Input: part model. Units: mm. Frame: model coordinates. A direction names the side the tool comes from. Give positions to 0.01 mm unless a question says otherwise; leave off trailing zeros. Order: outer loops, then holes, each group sorted by start corner. A loop starts at its lowest first (then second) coordinate and runs counter-clockwise, first axis right, second up. Notation, with made-up numbers: (15, 39.5) - (31, 39.5) arc R33 ccw to (31, 67.5) - close; hole circle Ø3 at (40, -6.75). An arc over 180 degrees is marked (long way). Answer in a Markdown table with one row per item. Add a question column.
1. Mould query, pull axis Y, two halves, no side actions, for faces 3 (the face through (-2, 2, 0)), 4 (the face through (69.59, 102.26, -3.04)), 5 (the face through (-2, -130, -3)). Classes: released by +Y, released by -Y, zero draft, split by the parting line, or undercut.
2. Access query for faces 1 (the face through (-132.5, -2, -3)), 2 (the face through (75, 109.05, -3)). Directions: +Z, -Z, +X, -X, +Y, -Y. A direction counts if a zero-diameter tool reaches every point of the face in a straight line with its end or side. Return the directions, or none.
3. Ray query, line 1 (X direction, y = -78, z = -3.65) (3 decimals); line 2 (Y direction, x = -99.65, z = -3.5); line 3 (Y direction, x = -49, z = -5.2). Return the intervals inside material, ascending. Write a range as [from, to].
4. Section query B-B on z = -3.25. Count the separate pieces of the cut face and the enclosed holes in it, and give its area (3 significant figures).
5. Section query A-A on x = -99.65. Return loops of the section in (y, z).
```python
from build123d import *

# Parameters (mm, degrees)
CROQUIS1_W                        = 265
CROQUIS1_H                        = 260
BRIDA_BASE1_DEPTH                 = 6
TALADRO_DE_MARGEN_PARA_M181_D     = 20
DI_METRO_DE_TALADRO_16_0_16_1_D   = 16
RANURA_START                      = -6
RANURA_DE_MARGEN_PARA_M3_54_DEPTH = 6
TALADRO_DE_MARGEN_PARA_M31_D      = 3.75
CORTAR_EXTRUIR1_DEPTH             = 186.72089274
CORTAR_EXTRUIR1_DEPTH_BACK        = 186.72089274
CROQUIS23_R                       = 1.875
CORTAR_EXTRUIR3_DEPTH             = 186.72089274
CORTAR_EXTRUIR3_DEPTH_BACK        = 186.72089274
CROQUIS29_R                       = 1.6
RANURA_DE_MARGEN_PARA_M61_DEPTH   = 6
TALADRO_DE_MARGEN_PARA_M32_D      = 3.4


# Read off the part's stored shape, not the designer's step: Ranura de margen para M3.54, Ranura de margen para M61
# Sheet-metal steps are written as plain solids
with BuildPart() as part:
    # Croquis1 → Brida base1 (new body)
    with BuildSketch(Plane.XY):
        Rectangle(CROQUIS1_W, CROQUIS1_H)
    extrude(amount=-BRIDA_BASE1_DEPTH)

    # Taladro de margen para M181 (through all)
    with Locations(Plane.XY):
        with Locations((62.219531128, 95.5), (-62.219531128, 95.5)):
            Hole(TALADRO_DE_MARGEN_PARA_M181_D / 2)

    # Diámetro de taladro Ø16.0 (16)1 (through all)
    with Locations(Plane(origin=(0, 0, -6), x_dir=(-1, 0, 0), z_dir=(0, 0, -1))):
        with Locations((-99.65, 100), (99.65, 100)):
            Hole(DI_METRO_DE_TALADRO_16_0_16_1_D / 2)

    # Ranura de margen para M3.54 outline → Ranura de margen para M3.54 (cut)
    with BuildSketch(Plane.XY.offset(RANURA_START)):
        with BuildLine():
            ThreePointArc((52.769531128, 78.05), (54.719531128, 80), (52.769531128, 81.95))
            Line((52.769531128, 81.95), (46.669531128, 81.95))
            ThreePointArc((46.669531128, 81.95), (44.719531128, 80), (46.669531128, 78.05))
            Line((46.669531128, 78.05), (52.769531128, 78.05))
        make_face()
        with BuildLine():
            ThreePointArc((71.669531128, 81.95), (69.719531128, 80), (71.669531128, 78.05))
            Line((71.669531128, 78.05), (77.769531128, 78.05))
            ThreePointArc((77.769531128, 78.05), (79.719531128, 80), (77.769531128, 81.95))
            Line((77.769531128, 81.95), (71.669531128, 81.95))
        make_face()
        with BuildLine():
            ThreePointArc((-77.769531128, 81.95), (-79.719531128, 80), (-77.769531128, 78.05))
            Line((-77.769531128, 78.05), (-71.669531128, 78.05))
            ThreePointArc((-71.669531128, 78.05), (-69.719531128, 80), (-71.669531128, 81.95))
            Line((-71.669531128, 81.95), (-77.769531128, 81.95))
        make_face()
        with BuildLine():
            ThreePointArc((-52.769531128, 81.95), (-54.719531128, 80), (-52.769531128, 78.05))
            Line((-52.769531128, 78.05), (-46.669531128, 78.05))
            ThreePointArc((-46.669531128, 78.05), (-44.719531128, 80), (-46.669531128, 81.95))
            Line((-46.669531128, 81.95), (-52.769531128, 81.95))
        make_face()
        with BuildLine():
            ThreePointArc((77.769531128, 109.05), (79.719531128, 111), (77.769531128, 112.95))
            Line((77.769531128, 112.95), (71.669531128, 112.95))
            ThreePointArc((71.669531128, 112.95), (69.719531128, 111), (71.669531128, 109.05))
            Line((71.669531128, 109.05), (77.769531128, 109.05))
        make_face()
        with BuildLine():
            ThreePointArc((46.669531128, 112.95), (44.719531128, 111), (46.669531128, 109.05))
            Line((46.669531128, 109.05), (52.769531128, 109.05))
            ThreePointArc((52.769531128, 109.05), (54.719531128, 111), (52.769531128, 112.95))
            Line((52.769531128, 112.95), (46.669531128, 112.95))
        make_face()
        with BuildLine():
            ThreePointArc((-52.769531128, 112.95), (-54.719531128, 111), (-52.769531128, 109.05))
            Line((-52.769531128, 109.05), (-46.669531128, 109.05))
            ThreePointArc((-46.669531128, 109.05), (-44.719531128, 111), (-46.669531128, 112.95))
            Line((-46.669531128, 112.95), (-52.769531128, 112.95))
        make_face()
        with BuildLine():
            ThreePointArc((-77.769531128, 112.95), (-79.719531128, 111), (-77.769531128, 109.05))
            Line((-77.769531128, 109.05), (-71.669531128, 109.05))
            ThreePointArc((-71.669531128, 109.05), (-69.719531128, 111), (-71.669531128, 112.95))
            Line((-71.669531128, 112.95), (-77.769531128, 112.95))
        make_face()
    extrude(amount=RANURA_DE_MARGEN_PARA_M3_54_DEPTH, mode=Mode.SUBTRACT)

    # Taladro de margen para M31 (through all)
    with Locations(Plane(origin=(0, 0, -6), x_dir=(-1, 0, 0), z_dir=(0, 0, -1))):
        with Locations((-93.405002002, 81), (-121.5, 91.02623214), (-93.5, 120.079280366)):
            taladro_de_margen_para_m31 = Hole(TALADRO_DE_MARGEN_PARA_M31_D / 2)

    # Simetría1: Taladro de margen para M31 across plane
    add(taladro_de_margen_para_m31.mirror(Plane(origin=(0, 0, 0), x_dir=(0, 0, 1), z_dir=(1, 0, 0))), mode=Mode.SUBTRACT)

    # Croquis23 → Cortar-Extruir1 (cut, two sides: drawn at the far end of the back side and taken through both)
    with BuildSketch(Plane.XY.offset(-CORTAR_EXTRUIR1_DEPTH_BACK)):
        with Locations((-119.5, -70)):
            Circle(CROQUIS23_R)
        with Locations((-119.5, -78)):
            Circle(CROQUIS23_R)
        with Locations((119.5, -78)):
            Circle(CROQUIS23_R)
        with Locations((119.5, -70)):
            Circle(CROQUIS23_R)
    extrude(amount=CORTAR_EXTRUIR1_DEPTH + CORTAR_EXTRUIR1_DEPTH_BACK, mode=Mode.SUBTRACT)

    # Croquis29 → Cortar-Extruir3 (cut, two sides: drawn at the far end of the back side and taken through both)
    with BuildSketch(Plane(origin=(0, 0, -6), x_dir=(-1, 0, 0), z_dir=(0, 0, -1)).offset(-CORTAR_EXTRUIR3_DEPTH_BACK)):
        with Locations((24.13, -110)):
            Circle(CROQUIS29_R)
        with Locations((-24.13, -108.73)):
            Circle(CROQUIS29_R)
        with Locations((24.13, -27.45)):
            Circle(CROQUIS29_R)
    extrude(amount=CORTAR_EXTRUIR3_DEPTH + CORTAR_EXTRUIR3_DEPTH_BACK, mode=Mode.SUBTRACT)

    # Ranura de margen para M61 outline → Ranura de margen para M61 (cut)
    with BuildSketch(Plane.XY.offset(RANURA_START)):
        with BuildLine():
            ThreePointArc((-118, 118), (-114.5, 121.5), (-118, 125))
            Line((-118, 125), (-121, 125))
            ThreePointArc((-121, 125), (-124.5, 121.5), (-121, 118))
            Line((-121, 118), (-118, 118))
        make_face()
        with BuildLine():
            ThreePointArc((118, 125), (114.5, 121.5), (118, 118))
            Line((118, 118), (121, 118))
            ThreePointArc((121, 118), (124.5, 121.5), (121, 125))
            Line((121, 125), (118, 125))
        make_face()
        with BuildLine():
            ThreePointArc((121, -125), (124.5, -121.5), (121, -118))
            Line((121, -118), (118, -118))
            ThreePointArc((118, -118), (114.5, -121.5), (118, -125))
            Line((118, -125), (121, -125))
        make_face()
        with BuildLine():
            ThreePointArc((-121, -118), (-124.5, -121.5), (-121, -125))
            Line((-121, -125), (-118, -125))
            ThreePointArc((-118, -125), (-114.5, -121.5), (-118, -118))
            Line((-118, -118), (-121, -118))
        make_face()
    extrude(amount=RANURA_DE_MARGEN_PARA_M61_DEPTH, mode=Mode.SUBTRACT)

    # Taladro de margen para M32 (through all)
    with Locations(Plane(origin=(0, 0, -6), x_dir=(-1, 0, 0), z_dir=(0, 0, -1))):
        with Locations((60, 125), (0, 125), (-60, 125)):
            Hole(TALADRO_DE_MARGEN_PARA_M32_D / 2)


solid = part.part
```
Answer:
| question | item | result |
|---|---|---|
| 1 | face 3 | zero draft |
| 1 | face 4 | undercut |
| 1 | face 5 | released by -Y |
| 2 | face 1 | +Z, -Z, -X, +Y, -Y |
| 2 | face 2 | +Z, -Z |
| 3 | line 1 | x = [-132.5, -121.375], [-117.625, 117.625], [121.375, 132.5] |
| 3 | line 2 | y = [-130, 92], [108, 130] |
| 3 | line 3 | y = [-130, 78.05], [81.95, 109.05], [112.95, 130] |
| 4 | separate pieces | 1 |
| 4 | enclosed holes | 32 |
| 4 | area | 67,200 mm² |
| 5 | outline | (-130, -6) - (92, -6) - (92, 0) - (-130, 0) - close; (108, -6) - (130, -6) - (130, 0) - (108, 0) - close |
